Print and shaded views of the part. All mm, measured from the part's lowest x, y and z. A direction names the side the tool comes from. Round coordinates to 2 decimals unless told otherwise and drop trailing zeros. Loops run counter-clockwise (first coordinate to the right, second up) from the corner with the lowest first, then second, coordinate; pieces in that order, holes last. Notation, with made-up numbers: (-3, 6.25) -> (37, 6.25) arc R24 ccw to (37, 33.25) -> close; hole circle Ø6 at (1, 62.25). An arc over 180 degrees is marked (long way). Use a Markdown table: item, result.
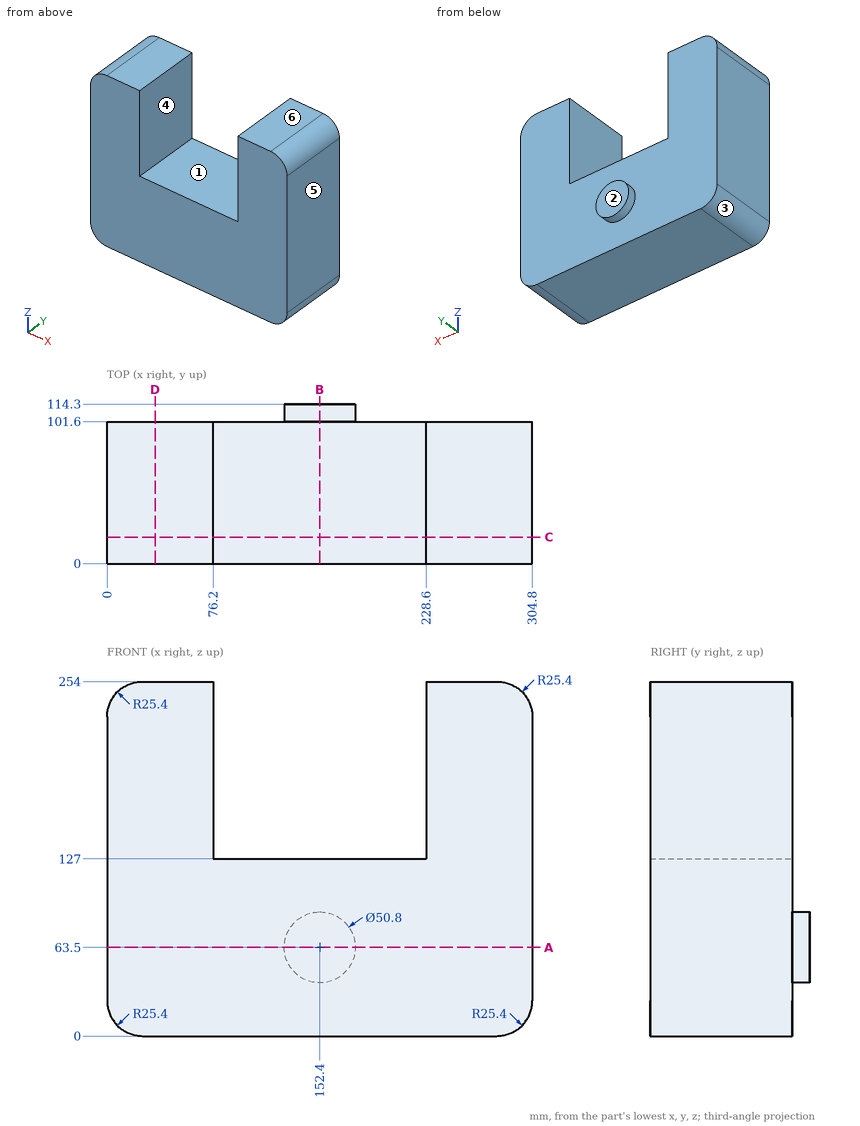
Q1. Band-saw the part on D-D, the plane x = 34.5. Give the cut face in (y, z), plus the area to 3 significant figures.
Results list:
| item | result |
|---|---|
| outline | (0, 0) -> (101.6, 0) -> (101.6, 254) -> (0, 254) -> close |
| area | 25,800 mm² |
Q2. Flat gauge pins, fed straight in: pin 1 (10 mm diameter, centred on x = 250, z = 68.5, fed in from +Y); pin 2 (4 mm diameter, centred on x = 216, y = 28.5, fed in from +Z). Where does each tip first touch, or does it go through?
Results list:
| item | result |
|---|---|
| pin 1 | stops at y = 101.6 |
| pin 2 | stops at z = 127 |
Q3. Band-saw the part on C-C, the plane y = 19. Give the cut face in (x, z), plus the area to 3 significant figures.
Results list:
| item | result |
|---|---|
| outline | (0, 25.4) arc R25.4 ccw to (25.4, 0) -> (279.4, 0) arc R25.4 ccw to (304.8, 25.4) -> (304.8, 228.6) arc R25.4 ccw to (279.4, 254) -> (228.6, 254) -> (228.6, 127) -> (76.2, 127) -> (76.2, 254) -> (25.4, 254) arc R25.4 ccw to (0, 228.6) -> close |
| area | 57,500 mm² |
Q4. Pull direction X, two halves, no side cores. Call the marked faces 3, 4, 5 and 6: released by +X, released by -X, zero draft, split by the parting line, or undercut.
Results list:
| item | result |
|---|---|
| face 3 | released by -X |
| face 4 | undercut |
| face 5 | released by +X |
| face 6 | zero draft |
Q5. Tool access for the marked faces 1 and 2: list every direction of +Z, -Z, +X, -X, +Y, -Y with a clear straight run to the whole face (end or side of a thin tool).
Results list:
| item | result |
|---|---|
| face 1 | +Z, +Y, -Y |
| face 2 | +Z, -Z, +X, -X, +Y |
Q6. Band-saw the part on A-A, the plane z = 63.5. Give the cut face in (x, y), plus the area to 3 significant figures.
Results list:
| item | result |
|---|---|
| outline | (0, 0) -> (304.8, 0) -> (304.8, 101.6) -> (177.8, 101.6) -> (177.8, 114.3) -> (127, 114.3) -> (127, 101.6) -> (0, 101.6) -> close |
| area | 31,600 mm² |
Q7. Drill centre lines: L1, parallel to X at y = 59.5, z = 169.5; L2, parallel to Z at x = 221.5, y = 71; L3, parallel to Y at x = 64, z = 232. Where is each one in solid material? Low to high. Write a range as from..to.
Results list:
| item | result |
|---|---|
| L1 | x = 0..76.2, 228.6..304.8 |
| L2 | z = 0..127 |
| L3 | y = 0..101.6 |
Q8. Band-saw the part on B-B, the plane x = 152.4. Give the cut face in (y, z), plus the area to 3 significant figures.
Results list:
| item | result |
|---|---|
| outline | (0, 0) -> (101.6, 0) -> (101.6, 38.1) -> (114.3, 38.1) -> (114.3, 88.9) -> (101.6, 88.9) -> (101.6, 127) -> (0, 127) -> close |
| area | 13,500 mm² |
